Geometry check sheet. Reference: drawing and pictorial views, mm from the part's lowest x, y, z. A direction names the side the tool comes from. Give positions to 0.01 mm unless a question says otherwise; leave off trailing zeros. Write each loop counter-clockwise with the first axis right and the second up, starting at its lowest first coordinate (ties: lowest second). Pieces come first, ordered by that corner, then holes. Notation, with made-up numbers: (36.25, -38.5) -> (76.25, -38.5) arc R8 ccw to (76.25, -33.5) -> close; hole circle Ø6 at (-3, -36). An arc over 180 degrees is marked (long way). Use a Markdown table: item, result. Add a question column.
1. Release check for a two-part mould opening along X. For the marked faces 1, 2, 3 and 4 record: released by +X, released by -X, zero draft, split by the parting line, or undercut.
2. Cross-section at C-C (x = 9.85). Count the separate pieces of the cut face and the enclosed holes in it, then the cut area to 4 significant figures.
3. Cross-section at D-D (z = 1.75). Enter the section's corners in (x, y).
4. Cross-section at A-A (x = 16.35). Enter the section's corners in (y, z), then the cut area to 3 significant figures.
5. Set-up check for the marked faces 5 and 6: record each of +Z, -Z, +X, -X, +Y, -Y from which the full face is reachable in a straight line by a thin tool's end or side.
6. Scan lines: probe 1 along Y at (x, z) = (9.75, 3.85); probe 2 along X at (y, z) = (11, 2.4); probe 3 along Z at (x, y) = (5.5, 15.5). Record each from-to range of solid material in increasing order. Write a range as [from, to].
7. Gauge pin test, flat ends, axial feed: P1, Ø2, axis at x = 3.5, z = 2, coming from the -Y side; P2, Ø1.8, axis at x = 10, y = 9, coming from the +Z side; P3, Ø1.2, axis at x = 9.85, y = 9.85, coming from the -Z side; P4, Ø1, axis at x = 3.5, y = 15.5, coming from the +Z side. Record the tip position at first contact, or that the pin passes through.
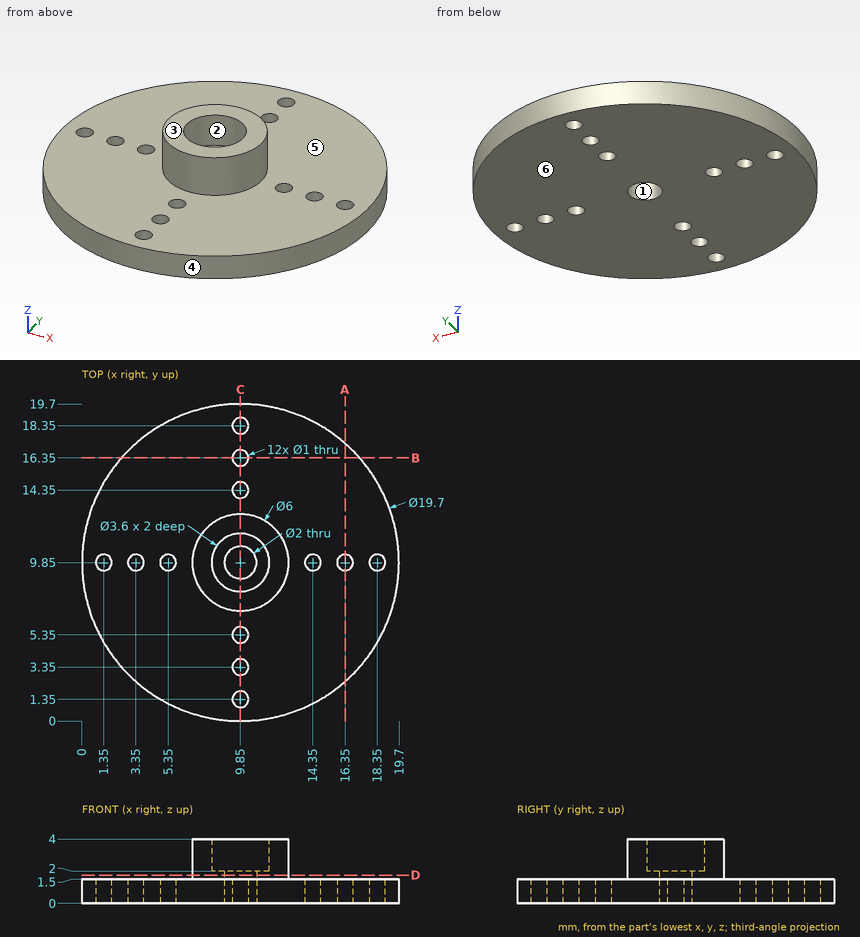
Worked answers:
| question | item | result |
|---|---|---|
| 1 | face 1 | undercut |
| 1 | face 2 | undercut |
| 1 | face 3 | zero draft |
| 1 | face 4 | split by the parting line |
| 2 | separate pieces | 8 |
| 2 | enclosed holes | 0 |
| 2 | area | 24.35 mm² |
| 3 | outline | circle Ø6 at (9.85, 9.85); hole circle Ø2 at (9.85, 9.85) |
| 4 | outline | (2.45, 0) -> (9.35, 0) -> (9.35, 1.5) -> (2.45, 1.5) -> close; (10.35, 0) -> (17.25, 0) -> (17.25, 1.5) -> (10.35, 1.5) -> close |
| 4 | area | 20.7 mm² |
| 5 | face 5 | +Z |
| 5 | face 6 | -Z, +X, -X, +Y, -Y |
| 6 | probe 1 | y = [6.85, 8.05], [11.65, 12.85] |
| 6 | probe 2 | x = [7.08, 8.47], [11.23, 12.62] |
| 6 | probe 3 | z = [0, 1.5] |
| 7 | P1 | stops at y = 1.67 |
| 7 | P2 | stops at z = 2 |
| 7 | P3 | passes through |
| 7 | P4 | stops at z = 1.5 |
